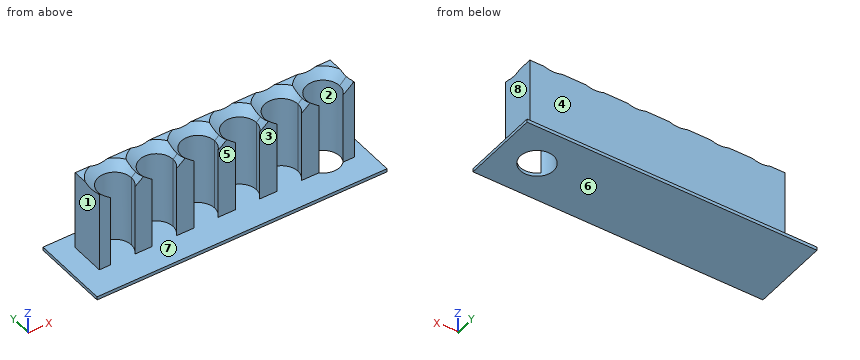
```python
from build123d import *

# Parameters (mm, degrees)
F1_DEPTH     = 50
F0_W         = 174.0209832788
F0_H         = 46.8094409443
F2_DEPTH     = 2
F3_T2_ANGLE  = 297.2148412711
F3_T4_ANGLE  = 297.2148412711
F3_T6_ANGLE  = 297.2148412711
F3_T8_ANGLE  = 297.2148412711
F3_T10_ANGLE = 297.2148412711
F3_T12_ANGLE = 297.2148412711
F3_T14_ANGLE = 117.0391625113
F3_T16_ANGLE = 117.0391625113
F3_T18_ANGLE = 117.0391625113
F3_T20_ANGLE = 117.0391625113
F3_T22_ANGLE = 117.0391625113
F3_T24_ANGLE = 117.0391625113


# Not quite as in the source:
# - a fillet or chamfer that OpenCascade refuses, or shapes differently, is made with other operations: its cross-section is extruded or revolved along the edge and cut away or added


with BuildPart() as f1:
    # F0 (on Top) → F1 (new body)
    with BuildSketch(Plane.XY):
        with BuildLine():
            ThreePointArc((-63.3511276029, 24.1111628711), (-59.7746098829, 40.2694854105), (-46.0804665685, 30.9768375009))
            ThreePointArc((-46.0804665685, 30.9768375009), (-46.7878186589, 27.2826941865), (-48.809805534, 24.1111628711))
            Line((-48.809805534, 24.1111628711), (-38.3511276029, 24.1111628711))
            ThreePointArc((-38.3511276029, 24.1111628711), (-34.7746098829, 40.2694854105), (-21.0804665685, 30.9768375009))
            ThreePointArc((-21.0804665685, 30.9768375009), (-21.7878186589, 27.2826941865), (-23.809805534, 24.1111628711))
            Line((-23.809805534, 24.1111628711), (-13.3511276029, 24.1111628711))
            ThreePointArc((-13.3511276029, 24.1111628711), (-9.7746098829, 40.2694854105), (3.9195334315, 30.9768375009))
            ThreePointArc((3.9195334315, 30.9768375009), (3.2121813411, 27.2826941865), (1.190194466, 24.1111628711))
            Line((1.190194466, 24.1111628711), (11.6488723971, 24.1111628711))
            ThreePointArc((11.6488723971, 24.1111628711), (15.2253901171, 40.2694854105), (28.9195334315, 30.9768375009))
            ThreePointArc((28.9195334315, 30.9768375009), (28.2121813411, 27.2826941865), (26.190194466, 24.1111628711))
            Line((26.190194466, 24.1111628711), (36.6488723971, 24.1111628711))
            ThreePointArc((36.6488723971, 24.1111628711), (40.2253901171, 40.2694854105), (53.9195334315, 30.9768375009))
            ThreePointArc((53.9195334315, 30.9768375009), (53.2121813411, 27.2826941865), (51.190194466, 24.1111628711))
            Line((51.190194466, 24.1111628711), (61.6488723971, 24.1111628711))
            ThreePointArc((61.6488723971, 24.1111628711), (65.2253901171, 40.2694854105), (78.9195334315, 30.9768375009))
            ThreePointArc((78.9195334315, 30.9768375009), (78.2121813411, 27.2826941865), (76.190194466, 24.1111628711))
            Line((76.190194466, 24.1111628711), (82.9195334315, 24.1111628711))
            Line((82.9195334315, 24.1111628711), (82.9195334315, 44.9768375009))
            Line((82.9195334315, 44.9768375009), (-70.0804665685, 44.9768375009))
            Line((-70.0804665685, 44.9768375009), (-70.0804665685, 24.1111628711))
            Line((-70.0804665685, 24.1111628711), (-63.3511276029, 24.1111628711))
        make_face()
    extrude(amount=F1_DEPTH)

    # F0 (on Top) → F2 (join)
    with BuildSketch(Plane.XY):
        with Locations((4.097443074, 30.9768363368)):
            Rectangle(F0_W, F0_H)
        Polygon((-70.0804665685, 16.9768375009), (-70.0804665685, 24.1111628711), (-70.0804665685, 44.9768375009), (82.9195334315, 44.9768375009), (82.9195334315, 24.1111628711), (82.9195334315, 16.9768375009), align=None, mode=Mode.SUBTRACT)
        with BuildLine():
            ThreePointArc((-48.809805534, 24.1111628711), (-56.0804665685, 20.9768375009), (-63.3511276029, 24.1111628711))
            Line((-63.3511276029, 24.1111628711), (-70.0804665685, 24.1111628711))
            Line((-70.0804665685, 24.1111628711), (-70.0804665685, 16.9768375009))
            Line((-70.0804665685, 16.9768375009), (82.9195334315, 16.9768375009))
            Line((82.9195334315, 16.9768375009), (82.9195334315, 24.1111628711))
            Line((82.9195334315, 24.1111628711), (76.190194466, 24.1111628711))
            ThreePointArc((76.190194466, 24.1111628711), (68.9195334315, 20.9768375009), (61.6488723971, 24.1111628711))
            Line((61.6488723971, 24.1111628711), (51.190194466, 24.1111628711))
            ThreePointArc((51.190194466, 24.1111628711), (43.9195334315, 20.9768375009), (36.6488723971, 24.1111628711))
            Line((36.6488723971, 24.1111628711), (26.190194466, 24.1111628711))
            ThreePointArc((26.190194466, 24.1111628711), (18.9195334315, 20.9768375009), (11.6488723971, 24.1111628711))
            Line((11.6488723971, 24.1111628711), (1.190194466, 24.1111628711))
            ThreePointArc((1.190194466, 24.1111628711), (-6.0804665685, 20.9768375009), (-13.3511276029, 24.1111628711))
            Line((-13.3511276029, 24.1111628711), (-23.809805534, 24.1111628711))
            ThreePointArc((-23.809805534, 24.1111628711), (-31.0804665685, 20.9768375009), (-38.3511276029, 24.1111628711))
            Line((-38.3511276029, 24.1111628711), (-48.809805534, 24.1111628711))
        make_face()
        with BuildLine():
            ThreePointArc((-48.809805534, 24.1111628711), (-46.7878186589, 27.2826941865), (-46.0804665685, 30.9768375009))
            ThreePointArc((-46.0804665685, 30.9768375009), (-59.7746098829, 40.2694854105), (-63.3511276029, 24.1111628711))
            Line((-63.3511276029, 24.1111628711), (-48.809805534, 24.1111628711))
        make_face()
        with BuildLine():
            Line((-48.809805534, 24.1111628711), (-63.3511276029, 24.1111628711))
            ThreePointArc((-63.3511276029, 24.1111628711), (-56.0804665685, 20.9768375009), (-48.809805534, 24.1111628711))
        make_face()
        with BuildLine():
            ThreePointArc((-21.0804665685, 30.9768375009), (-34.7746098829, 40.2694854105), (-38.3511276029, 24.1111628711))
            Line((-38.3511276029, 24.1111628711), (-23.809805534, 24.1111628711))
            ThreePointArc((-23.809805534, 24.1111628711), (-21.7878186589, 27.2826941865), (-21.0804665685, 30.9768375009))
        make_face()
        with BuildLine():
            Line((-23.809805534, 24.1111628711), (-38.3511276029, 24.1111628711))
            ThreePointArc((-38.3511276029, 24.1111628711), (-31.0804665685, 20.9768375009), (-23.809805534, 24.1111628711))
        make_face()
        with BuildLine():
            ThreePointArc((3.9195334315, 30.9768375009), (-9.7746098829, 40.2694854105), (-13.3511276029, 24.1111628711))
            Line((-13.3511276029, 24.1111628711), (1.190194466, 24.1111628711))
            ThreePointArc((1.190194466, 24.1111628711), (3.2121813411, 27.2826941865), (3.9195334315, 30.9768375009))
        make_face()
        with BuildLine():
            Line((1.190194466, 24.1111628711), (-13.3511276029, 24.1111628711))
            ThreePointArc((-13.3511276029, 24.1111628711), (-6.0804665685, 20.9768375009), (1.190194466, 24.1111628711))
        make_face()
        with BuildLine():
            ThreePointArc((28.9195334315, 30.9768375009), (15.2253901171, 40.2694854105), (11.6488723971, 24.1111628711))
            Line((11.6488723971, 24.1111628711), (26.190194466, 24.1111628711))
            ThreePointArc((26.190194466, 24.1111628711), (28.2121813411, 27.2826941865), (28.9195334315, 30.9768375009))
        make_face()
        with BuildLine():
            Line((26.190194466, 24.1111628711), (11.6488723971, 24.1111628711))
            ThreePointArc((11.6488723971, 24.1111628711), (18.9195334315, 20.9768375009), (26.190194466, 24.1111628711))
        make_face()
        with BuildLine():
            Line((36.6488723971, 24.1111628711), (51.190194466, 24.1111628711))
            ThreePointArc((51.190194466, 24.1111628711), (53.2121813411, 27.2826941865), (53.9195334315, 30.9768375009))
            ThreePointArc((53.9195334315, 30.9768375009), (40.2253901171, 40.2694854105), (36.6488723971, 24.1111628711))
        make_face()
        with BuildLine():
            ThreePointArc((36.6488723971, 24.1111628711), (43.9195334315, 20.9768375009), (51.190194466, 24.1111628711))
            Line((51.190194466, 24.1111628711), (36.6488723971, 24.1111628711))
        make_face()
    extrude(amount=F2_DEPTH)

    # F3: chamfer of 5 on 6 edges, made by hand

    # F3_s1 → F3_t2 (revolve, cut)
    with BuildSketch(Plane(origin=(-31.7529692139, -16.3292082814, 0), x_dir=(0, 0, 1), z_dir=(0.8892979418, 0.4573282964, 0))):
        Polygon((45, -43.1948220704), (50, -38.1948220704), (50, -43.1948220704), align=None)
    revolve(axis=Axis((-56.0804665685, 30.9768375009, 50), (0, 0, -1)), revolution_arc=F3_T2_ANGLE, mode=Mode.SUBTRACT)

    # F3_s3 → F3_t4 (revolve, cut)
    with BuildSketch(Plane(origin=(-11.981698481, -6.1616804635, 0), x_dir=(0, 0, 1), z_dir=(0.8892979418, 0.4573282964, 0))):
        Polygon((45, -31.7616146605), (50, -26.7616146605), (50, -31.7616146605), align=None)
    revolve(axis=Axis((-31.0804665685, 30.9768375009, 50), (0, 0, -1)), revolution_arc=F3_T4_ANGLE, mode=Mode.SUBTRACT)

    # F3_s5 → F3_t6 (revolve, cut)
    with BuildSketch(Plane(origin=(7.7895722518, 4.0058473545, 0), x_dir=(0, 0, 1), z_dir=(0.8892979418, 0.4573282964, 0))):
        Polygon((45, -20.3284072505), (50, -15.3284072505), (50, -20.3284072505), align=None)
    revolve(axis=Axis((-6.0804665685, 30.9768375009, 50), (0, 0, -1)), revolution_arc=F3_T6_ANGLE, mode=Mode.SUBTRACT)

    # F3_s7 → F3_t8 (revolve, cut)
    with BuildSketch(Plane(origin=(27.5608429847, 14.1733751725, 0), x_dir=(0, 0, 1), z_dir=(0.8892979418, 0.4573282964, 0))):
        Polygon((45, -8.8951998406), (50, -3.8951998406), (50, -8.8951998406), align=None)
    revolve(axis=Axis((18.9195334315, 30.9768375009, 50), (0, 0, -1)), revolution_arc=F3_T8_ANGLE, mode=Mode.SUBTRACT)

    # F3_s9 → F3_t10 (revolve, cut)
    with BuildSketch(Plane(origin=(47.3321137176, 24.3409029904, 0), x_dir=(0, 0, 1), z_dir=(0.8892979418, 0.4573282964, 0))):
        Polygon((45, 2.5380075693), (50, 7.5380075693), (50, 2.5380075693), align=None)
    revolve(axis=Axis((43.9195334315, 30.9768375009, 50), (0, 0, -1)), revolution_arc=F3_T10_ANGLE, mode=Mode.SUBTRACT)

    # F3_s11 → F3_t12 (revolve, cut)
    with BuildSketch(Plane(origin=(67.1033844505, 34.5084308084, 0), x_dir=(0, 0, 1), z_dir=(0.8892979418, 0.4573282964, 0))):
        Polygon((45, 13.9712149792), (50, 18.9712149792), (50, 13.9712149792), align=None)
    revolve(axis=Axis((68.9195334315, 30.9768375009, 50), (0, 0, -1)), revolution_arc=F3_T12_ANGLE, mode=Mode.SUBTRACT)

    # F3_s13 → F3_t14 (revolve, cut)
    with BuildSketch(Plane.XZ.offset(-30.9768375009)):
        Polygon((78.9195334315, 45), (83.9195334315, 50), (78.9195334315, 50), align=None)
    revolve(axis=Axis((68.9195334315, 30.9768375009, 50), (0, 0, -1)), revolution_arc=F3_T14_ANGLE, mode=Mode.SUBTRACT)

    # F3_s15 → F3_t16 (revolve, cut)
    with BuildSketch(Plane.XZ.offset(-30.9768375009)):
        Polygon((53.9195334315, 45), (58.9195334315, 50), (53.9195334315, 50), align=None)
    revolve(axis=Axis((43.9195334315, 30.9768375009, 50), (0, 0, -1)), revolution_arc=F3_T16_ANGLE, mode=Mode.SUBTRACT)

    # F3_s17 → F3_t18 (revolve, cut)
    with BuildSketch(Plane.XZ.offset(-30.9768375009)):
        Polygon((28.9195334315, 45), (33.9195334315, 50), (28.9195334315, 50), align=None)
    revolve(axis=Axis((18.9195334315, 30.9768375009, 50), (0, 0, -1)), revolution_arc=F3_T18_ANGLE, mode=Mode.SUBTRACT)

    # F3_s19 → F3_t20 (revolve, cut)
    with BuildSketch(Plane.XZ.offset(-30.9768375009)):
        Polygon((3.9195334315, 45), (8.9195334315, 50), (3.9195334315, 50), align=None)
    revolve(axis=Axis((-6.0804665685, 30.9768375009, 50), (0, 0, -1)), revolution_arc=F3_T20_ANGLE, mode=Mode.SUBTRACT)

    # F3_s21 → F3_t22 (revolve, cut)
    with BuildSketch(Plane.XZ.offset(-30.9768375009)):
        Polygon((-21.0804665685, 45), (-16.0804665685, 50), (-21.0804665685, 50), align=None)
    revolve(axis=Axis((-31.0804665685, 30.9768375009, 50), (0, 0, -1)), revolution_arc=F3_T22_ANGLE, mode=Mode.SUBTRACT)

    # F3_s23 → F3_t24 (revolve, cut)
    with BuildSketch(Plane.XZ.offset(-30.9768375009)):
        Polygon((-46.0804665685, 45), (-41.0804665685, 50), (-46.0804665685, 50), align=None)
    revolve(axis=Axis((-56.0804665685, 30.9768375009, 50), (0, 0, -1)), revolution_arc=F3_T24_ANGLE, mode=Mode.SUBTRACT)


solid = f1.part
```
Build history of the part. All positions in model axes, mm. Face numbers are marked on the shaded views. A direction names the side the tool comes from. Round coordinates to 2 decimals unless told otherwise and drop trailing zeros. Write each loop counter-clockwise with the first axis right and the second up, starting at its lowest first coordinate (ties: lowest second). Pieces come first, ordered by that corner, then holes. Notation, with made-up numbers: (-39, 22) - (-4, 22) arc R38 cw to (-4, 60) - close; hole circle Ø4 at (27, 30.5). An arc over 180 degrees is marked (long way). Write each question's results on one line, items separated by ' | '. Start each with the question number.
Item 1: Mould opens along Y. For the marked faces 1, 2 and 3 say: pulls with the +Y half, pulls with the -Y half, needs draft (parallel to the pull), parting line crosses it, or undercut.
Item 2: Saw through at A-A (z = 21). Write the cut outline in (x, y), and give its area (3 significant figures).
Item 3: Wall check: L1, parallel to Z at x = -5.5, y = 50; L2, parallel to Y at x = 30.5, z = 26; L3, parallel to X at y = 43, z = 45.5. Give the ranges that are in metal, low to high. Write a range as [from, to].
Item 4: Saw through at B-B (y = 15.5). Write the cut outline in (x, z), and give its area (3 significant figures).
Item 5: Which spindle directions (+Z, -Z, +X, -X, +Y, -Y) get a long thin tool onto all of the face, cutting with end or side? Do the marked faces 4, 5, 6, 7 and 8. Say none if no direction does.
Item 6: Drop flat-ended pins along their axis: P1, Ø11.5, axis at x = -18, z = 30.5, coming from the -Y side; P2, Ø5, axis at x = 53, z = 21.5, coming from the +Y side; P3, Ø5, axis at y = 36.5, z = 29.5, coming from the -X side. Give the stop position or say it passes through.
Results are:
1) face 1: needs draft | face 2: undercut | face 3: pulls with the -Y half
2) outline: (-70.08, 24.11) - (-63.35, 24.11) arc R10 cw (long way) to (-48.81, 24.11) - (-38.35, 24.11) arc R10 cw (long way) to (-23.81, 24.11) - (-13.35, 24.11) arc R10 cw (long way) to (1.19, 24.11) - (11.65, 24.11) arc R10 cw (long way) to (26.19, 24.11) - (36.65, 24.11) arc R10 cw (long way) to (51.19, 24.11) - (61.65, 24.11) arc R10 cw (long way) to (76.19, 24.11) - (82.92, 24.11) - (82.92, 44.98) - (-70.08, 44.98) - close | area: 1,500 mm²
3) L1: z = [0, 2] | L2: y = [24.11, 44.98] | L3: x = [-70.08, 82.92]
4) outline: (-82.91, 0) - (91.11, 0) - (91.11, 2) - (-82.91, 2) - close | area: 348 mm²
5) face 4: +Z, +X, -X, +Y | face 5: +Z, +X, -X, -Y | face 6: -Z, +X, -X, +Y, -Y | face 7: +Z | face 8: +Z, +X, +Y, -Y
6) P1: stops at y = 24.11 | P2: stops at y = 44.98 | P3: stops at x = -70.08
